```python
from build123d import *

# Parameters (mm, degrees)
ESBO_O1_W                = 116
ESBO_O1_H                = 74
RESSALTO_EXTRUS_O1_DEPTH = 3
RESSALTO_EXTRUS_O2_DEPTH = 3
FILETE1_R                = 3


with BuildPart() as part:
    # Esboço1 → Ressalto-extrusão1 (new body)
    with BuildSketch(Plane.XY):
        Rectangle(ESBO_O1_W, ESBO_O1_H)
    extrude(amount=RESSALTO_EXTRUS_O1_DEPTH)

    # Esboço2 → Ressalto-extrusão2 (add)
    with BuildSketch(Plane.ZY.offset(58)):
        with BuildLine():
            Line((3, 34), (36, 34))
            ThreePointArc((36, 34), (43.071067812, 31.071067812), (46, 24))
            Line((46, 24), (46, -24))
            ThreePointArc((46, -24), (43.071067812, -31.071067812), (36, -34))
            Line((36, -34), (3, -34))
            Line((3, -34), (3, 34))
        make_face()
    extrude(amount=-RESSALTO_EXTRUS_O2_DEPTH)

    # Filete1
    filete1_edges = [part.edges().sort_by_distance(p)[0] for p in [
        (-55, 0, 3),
    ]]
    fillet(filete1_edges, radius=FILETE1_R)


solid = part.part
```
The model under review builds one solid part; all positions refer to its coordinate system, in mm. A direction names the side the tool comes from. Give positions to 0.01 mm unless a question says otherwise; leave off trailing zeros. Write each loop counter-clockwise with the first axis right and the second up, starting at its lowest first coordinate (ties: lowest second). Pieces come first, ordered by that corner, then holes. Notation, with made-up numbers: M 63.5,41 L 90.5,41 A17 cw 90.5,50 Z; hole C 83.5,80.5 d5. An arc over 180 degrees is marked long. Answer in a Markdown table with one row per item.
Item 1: Tool access review of faces 1 (the face through (-57, 0, 46)), 2 (the face through (-56, 34, 19)), 3 (the face through (-55, 0, 26)), 4 (the face through (-56, -34, 20)), 5 (the face through (-1, 37, 1)): name each direction out of +Z, -Z, +X, -X, +Y, -Y from which nothing blocks a thin tool from reaching the whole face with its end or side.
Check sheet entries:
| item | result |
|---|---|
| face 1 | +Z, +X, -X, +Y, -Y |
| face 2 | +Z, +X, -X, +Y |
| face 3 | +Z, +X, +Y, -Y |
| face 4 | +Z, +X, -X, -Y |
| face 5 | +Z, -Z, +X, -X, +Y |
Item 2: Add section B-B on x = -50.5. Give the boundary of the cut face in (y, z), plus the area to 3 significant figures.
Check sheet entries:
| item | result |
|---|---|
| outline | M -37,0 L 37,0 L 37,3 L -37,3 Z |
| area | 222 mm2 |
Item 3: For P1, Ø2, axis at x = -43, y = -10, coming from the +Z side; P2, Ø1.8, axis at x = -53.5, z = 24.5, coming from the +Y side; P3, Ø1, axis at y = -19.5, z = 18, coming from the +X side; P4, Ø3, axis at x = -56.5, z = 18.5, coming from the -Y side, all flat-tipped, find the tip position at first contact; note any pin that passes through.
Check sheet entries:
| item | result |
|---|---|
| P1 | z = 3 |
| P2 | through |
| P3 | x = -55 |
| P4 | y = -34 |
Item 4: For line 1 along X through (y, z) = (-9.5, 15); line 2 along Z through (x, y) = (-29.5, -9.5); line 3 along X through (y, z) = (26, 4.5), list the stretches that pass through material, from the lowest coordinate up.
Check sheet entries:
| item | result |
|---|---|
| line 1 | -58 to -55 |
| line 2 | 0 to 3 |
| line 3 | -58 to -54.6 |
Item 5: Add section D-D on y = -28. Give the boundary of the cut face in (x, z), plus the area to 3 significant figures.
Check sheet entries:
| item | result |
|---|---|
| outline | M -58,0 L 58,0 L 58,3 L -52,3 A3 cw -55,6 L -55,45.17 L -58,45.17 Z |
| area | 476 mm2 |
Item 6: Add section A-A on y = -14.5. Give the boundary of the cut face in (x, z).
Check sheet entries:
| item | result |
|---|---|
| outline | M -58,0 L 58,0 L 58,3 L -52,3 A3 cw -55,6 L -55,46 L -58,46 Z |
Item 7: Add section C-C on z = 8.5. Give the boundary of the cut face in (x, y), plus the area to 3 significant figures.
Check sheet entries:
| item | result |
|---|---|
| outline | M -58,-34 L -55,-34 L -55,34 L -58,34 Z |
| area | 204 mm2 |
